Source: CAD feature listing. Evaluate the final solid. Frame: model axes, mm. A direction names the side the tool comes from. Round coordinates to 2 decimals unless told otherwise and drop trailing zeros. Order: outer loops, then holes, each group sorted by start corner. A loop starts at its lowest first (then second) coordinate and runs counter-clockwise, first axis right, second up. Notation, with made-up numbers: M 12,15 L 42,15 A10 cw 42,20 Z; hole C -26,37.25 d11. An arc over 180 degrees is marked long. Answer as CSV lines item,"result". Start each with the question number.
Item 1: Section query C-C on z = 9. Return the cut outline in (x, y), plus the area to 3 significant figures.
Item 2: Pull-direction query (Z, two-part tool) for faces 4 (the face through (-12, 22, 10)), 5 (the face through (-12, -21, -25)), 6 (the face through (-12.03, 34.23, -0.29)); classes: +Z half, -Z half, draft (parallel to the pull), parting line (faces both ways), or undercut.
Item 3: First-contact query: P1, Ø3.5, axis at y = 32, z = 0, coming from the -X side; P2, Ø1, axis at x = -10.5, y = 16.5, coming from the -Z side. Flat tips, straight axial feed; report the tip coordinate or a pass-through.
Item 4: Set-up query: faces 1 (the face through (-12, 22, -10)), 2 (the face through (-12, 4, 17)), 3 (the face through (-14, -2, 0)). Return all of +Z, -Z, +X, -X, +Y, -Y with unobstructed straight access to the full face (end or side cutting, diameter ignored); none if empty.
Item 5: Line query: line 1 (Z direction, x = -12.35, y = 24); line 2 (Y direction, x = -11.55, z = -22.5); line 3 (Y direction, x = -12.1, z = -5.5). Output: solid intervals per line, ascending. Write a range as [from, to].
Item 6: Section query B-B on z = 0. Return the cut outline in (x, y).
Item 7: Section query A-A on y = 32. Return the cut outline in (x, z), plus the area to 3 significant figures.
Item 8: Section query D-D on x = -12.95. Return the cut outline in (y, z), plus the area to 3 significant figures.
from build123d import *

# Parameters (mm, degrees)
SKETCH1_W           = 28
SKETCH1_H           = 28
SKETCH1_W_2         = 20
SKETCH1_H_2         = 20
BOSS_EXTRUDE1_DEPTH = 40
SKETCH2_R           = 2.25
CUT_EXTRUDE1_DEPTH  = 30
SKETCH5_W           = 50
SKETCH5_H           = 50
SKETCH5_R           = 1.8
SKETCH5_R_2         = 15
BOSS_EXTRUDE2_DEPTH = 4
SKETCH6_W           = 24
SKETCH6_H           = 28
CUT_EXTRUDE2_DEPTH  = 40
SKETCH7_W           = 4
SKETCH7_H           = 36
CUT_EXTRUDE3_DEPTH  = 4


with BuildPart() as part:
    # Sketch1 → Boss-Extrude1 (new body)
    with BuildSketch(Plane(origin=(0, 0, 0), x_dir=(1, 0, 0), z_dir=(0, 1, 0))):
        Rectangle(SKETCH1_W, SKETCH1_H)
        Rectangle(SKETCH1_W_2, SKETCH1_H_2, mode=Mode.SUBTRACT)
    extrude(amount=BOSS_EXTRUDE1_DEPTH)

    # Sketch2 → Cut-Extrude1 (cut)
    with BuildSketch(Plane.ZY.offset(14)):
        with Locations((0, 32)):
            Circle(SKETCH2_R)
        with Locations((0, 16)):
            Circle(SKETCH2_R)
    extrude(amount=-CUT_EXTRUDE1_DEPTH, mode=Mode.SUBTRACT)

    # Sketch5 → Boss-Extrude2 (add)
    with BuildSketch(Plane.ZY.offset(14)):
        with Locations((0, -21)):
            Rectangle(SKETCH5_W, SKETCH5_H)
        with Locations((-15.499780644, -5.500219356)):
            Circle(SKETCH5_R, mode=Mode.SUBTRACT)
        with Locations((15.499780644, -5.500219356)):
            Circle(SKETCH5_R, mode=Mode.SUBTRACT)
        with Locations((15.499780644, -36.499780644)):
            Circle(SKETCH5_R, mode=Mode.SUBTRACT)
        with Locations((-15.499780644, -36.499780644)):
            Circle(SKETCH5_R, mode=Mode.SUBTRACT)
        with Locations((0, -21)):
            Circle(SKETCH5_R_2, mode=Mode.SUBTRACT)
    extrude(amount=-BOSS_EXTRUDE2_DEPTH)

    # Sketch6 → Cut-Extrude2 (cut)
    with BuildSketch(Plane.XZ):
        with Locations((2, 0)):
            Rectangle(SKETCH6_W, SKETCH6_H)
    extrude(amount=-CUT_EXTRUDE2_DEPTH, mode=Mode.SUBTRACT)

    # Sketch7 → Cut-Extrude3 (cut)
    with BuildSketch(Plane.ZY.offset(14)):
        with Locations((-12, 22)):
            Rectangle(SKETCH7_W, SKETCH7_H)
        with Locations((12, 22)):
            Rectangle(SKETCH7_W, SKETCH7_H)
    extrude(amount=-CUT_EXTRUDE3_DEPTH, mode=Mode.SUBTRACT)


solid = part.part
Results:
1,outline,"M -14,-46 L -10,-46 L -10,-33 L -14,-33 Z; M -14,-9 L -10,-9 L -10,40 L -14,40 Z"
1,area,"248 mm^2"
2,face 4,"+Z half"
2,face 5,"-Z half"
2,face 6,"undercut"
3,P1,"through"
3,P2,"z = -10"
4,face 1,"-Z, +X, -X, +Y"
4,face 2,"+Z, +X, -X, +Y"
4,face 3,"+Z, -Z, -X, +Y, -Y"
5,line 1,"[-10, 10]"
5,line 2,"[-46, 4]"
5,line 3,"[-46, -34.96], [-7.04, 40]"
6,outline,"M -14,-46 L -10,-46 L -10,-36 L -14,-36 Z; M -14,-6 L -10,-6 L -10,13.75 L -14,13.75 Z; M -14,18.25 L -10,18.25 L -10,29.75 L -14,29.75 Z; M -14,34.25 L -10,34.25 L -10,40 L -14,40 Z"
7,outline,"M -14,-10 L -10,-10 L -10,-2.25 L -14,-2.25 Z; M -14,2.25 L -10,2.25 L -10,10 L -14,10 Z"
7,area,"62.0 mm^2"
8,outline,"M -46,-25 L 4,-25 L 4,-10 L 40,-10 L 40,10 L 4,10 L 4,25 L -46,25 Z; hole C -36.5,-15.5 d3.6; hole C -36.5,15.5 d3.6; hole C -21,0 d30; hole C -5.5,-15.5 d3.6; hole C -5.5,15.5 d3.6; hole C 16,0 d4.5; hole C 32,0 d4.5"
8,area,"2,440 mm^2"
